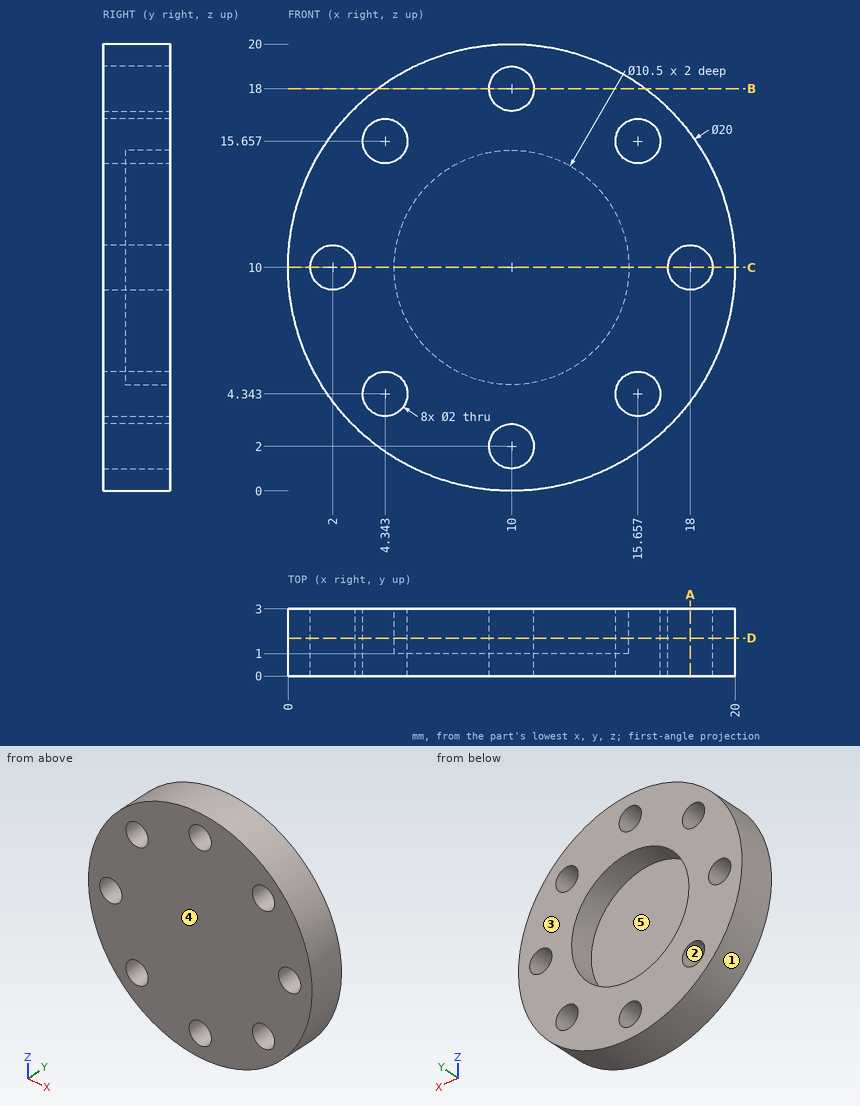
For this review, use the dimensioned drawing (mm, ordinates from the lowest corner) and the shaded views. A direction names the side the tool comes from. Round coordinates to 2 decimals unless told otherwise and drop trailing zeros. Write each loop counter-clockwise with the first axis right and the second up, starting at its lowest first coordinate (ties: lowest second). Pieces come first, ordered by that corner, then holes. Notation, with made-up numbers: (-28.5, 72) -> (-2.5, 72) arc R24 cw to (-2.5, 96) -> close; hole circle Ø2 at (-39.5, 34). An arc over 180 degrees is marked (long way). Use CSV: the item, a comma, the result in double quotes.
(1) Consider section B-B, the plane z = 18. Give the boundary of the cut face in (x, y).
Computed values:
outline,"(4, 0) -> (9, 0) -> (9, 3) -> (4, 3) -> close; (11, 0) -> (16, 0) -> (16, 3) -> (11, 3) -> close"
(2) To check wall thickness, follow L1, parallel to X at y = 2.1, z = 10; L2, parallel to X at y = 0.55, z = 4.5 (1 decimal); L3, parallel to X at y = 0.65, z = 9.5. State the ranges of each line that lie inside material, in increasing order. Write a range as [from, to].
Computed values:
L1,"[0, 1], [3, 4.75], [15.25, 17], [19, 20]"
L2,"[1.6, 3.4], [5.3, 14.7], [16.6, 18.4]"
L3,"[0.01, 1.13], [2.87, 17.13], [18.87, 19.99]"
(3) Consider section C-C, the plane z = 10. Give the boundary of the cut face in (x, y).
Computed values:
outline,"(0, 0) -> (1, 0) -> (1, 3) -> (0, 3) -> close; (3, 0) -> (17, 0) -> (17, 3) -> (15.25, 3) -> (15.25, 1) -> (4.75, 1) -> (4.75, 3) -> (3, 3) -> close; (19, 0) -> (20, 0) -> (20, 3) -> (19, 3) -> close"
(4) Draft analysis for pull direction X (two halves, no side actions). For the marked faces 1, 2 and 3, state which applies: +X half, -X half, draft (parallel to the pull), parting line (faces both ways), or undercut.
Computed values:
face 1,"parting line"
face 2,"undercut"
face 3,"draft"
(5) Clearance check with flat-ended pins moving along their axes: P1, Ø1, axis at x = 15, y = 0.5, coming from the +Z side; P2, Ø1.5, axis at y = 0.5, z = 3, coming from the -X side; P3, Ø1.6, axis at x = 15.66, z = 4.34, coming from the -Y side; P4, Ø3, axis at x = 9, z = 7.5, coming from the +Y side. State where each tip first meets the part, or that it passes through.
Computed values:
P1,"z = 18.93"
P2,"x = 2.19"
P3,"through"
P4,"y = 1"
(6) Consider section D-D, the plane y = 1.7. Give the number of separate pieces and of enclosed holes in the cut face, plus the area to 3 significant figures.
Computed values:
separate pieces,"1"
enclosed holes,"9"
area,"202 mm²"
(7) Consider section A-A, the plane x = 18. Give the boundary of the cut face in (y, z).
Computed values:
outline,"(0, 4) -> (3, 4) -> (3, 9) -> (0, 9) -> close; (0, 11) -> (3, 11) -> (3, 16) -> (0, 16) -> close"
(8) For the marked faces 4 and 5, list the 3-axis set-ups (+Z, -Z, +X, -X, +Y, -Y) from which the entire face can be reached by the end or side of a thin tool; tool diameter is ignored.
Computed values:
face 4,"+Z, -Z, +X, -X, -Y"
face 5,"+Y"
